from build123d import *

# Parameters (mm, degrees)
PAD012_DEPTH           = 5
LINEARPATTERN002_COUNT = 6
LINEARPATTERN002_PITCH = 15
SKETCH031_R            = 1.25
POCKET011_DEPTH        = 12
CHAMFER004_SIZE        = 1
FILLET004_R            = 3
FILLET005_R            = 1


with BuildPart() as part:
    # Sketch029 → Pad012 (new body, symmetric)
    with BuildSketch(Plane.YZ):
        Polygon((-18, 0), (93, 0), (85, 30), (-10, 30), align=None)
    extrude(amount=PAD012_DEPTH, both=True)

    # Sketch030 → Groove (revolve, cut)
    with BuildSketch(Plane.YZ):
        Polygon((0, 0), (1.8, 0), (1.8, 19.3), (2.5, 20), (2.5, 30), (0, 30), align=None)
    groove = revolve(axis=Axis((0, 0, 0), (0, 0, 1)), mode=Mode.SUBTRACT)

    # LinearPattern002: Groove ×6
    with Locations(*[(0, i * LINEARPATTERN002_PITCH, 0) for i in range(1, LINEARPATTERN002_COUNT)]):
        add(groove, mode=Mode.SUBTRACT)

    # Sketch031 → Pocket011 (cut)
    with BuildSketch(Plane.XY):
        with Locations((0, 85)):
            Circle(SKETCH031_R)
        with Locations((0, -10)):
            Circle(SKETCH031_R)
    extrude(amount=POCKET011_DEPTH, mode=Mode.SUBTRACT)

    # Chamfer004
    chamfer004_edges = [part.edges().sort_by_distance(p)[0] for p in [
        (0, -2.5, 30),
        (0, 12.5, 30),
        (0, 27.5, 30),
        (0, 42.5, 30),
        (0, 57.5, 30),
        (0, 72.5, 30),
    ]]
    chamfer(chamfer004_edges, length=CHAMFER004_SIZE)

    # Fillet004
    fillet004_edges = [part.edges().sort_by_distance(p)[0] for p in [
        (0, -10, 30),
        (0, 85, 30),
    ]]
    fillet(fillet004_edges, radius=FILLET004_R)

    # Fillet005
    fillet005_edges = [part.edges().sort_by_distance(p)[0] for p in [
        (5, -9.522873, 29.378967),
        (-5, 37.5, 30),
    ]]
    fillet(fillet005_edges, radius=FILLET005_R)


solid = part.part
Verification items for the finished model (mm, model axes). A direction names the side the tool comes from. Round coordinates to 2 decimals unless told otherwise and drop trailing zeros. Loops run counter-clockwise (first coordinate to the right, second up) from the corner with the lowest first, then second, coordinate; pieces in that order, holes last. Notation, with made-up numbers: (83, 81) - (106, 81) arc R23 cw to (106, 118) - close; hole circle Ø11 at (-37, 58). An arc over 180 degrees is marked (long way). Answer in a Markdown table with one row per item. Add a question column.
Q1. Section check B-B on z = 10. State how many separate pieces and enclosed holes the cut face has, plus the area to 3 significant figures.
Q2. Release check for a two-part mould opening along X. For faces 4 (the face through (0.056, -14.245, 14.081)), 5 (the face through (-4.7, 88.97, 14.01)), 6 (the face through (-0.1, 12.5, 24.6)), 7 (the face through (5, 37, 15)) record: pulls with the +X half, pulls with the -X half, needs draft (parallel to the pull), parting line crosses it, or undercut.
Q3. Material ranges on line 1 (X direction, y = 0, z = 19); line 2 (X direction, y = 60, z = 25.5); line 3 (Y direction, x = 3.5, z = 23), recorded low to high.
Q4. Gauge pin test, flat ends, axial feed: pin 1 (6 mm diameter, centred on x = 0, y = 30, fed in from +Z); pin 2 (4.5 mm diameter, centred on x = 0, y = 30, fed in from +Z); pin 3 (2 mm diameter, centred on x = -1, z = 12.5, fed in from -Y). Record the tip position at first contact, or that the pin passes through.
Q5. Section check A-A on y = 15. Enter the section's corners in (x, z), plus the area to 3 significant figures.
Q6. Tool access check on faces 1 (the face through (0.96, 47.31, 24.56)), 2 (the face through (0.672, -8.946, 5.916)), 3 (the face through (1.095, 73.572, 9.785)). Record the directions out of +Z, -Z, +X, -X, +Y, -Y that give a thin tool (end or side, any length) a straight path to the whole face; none if there is none.
Found:
| question | item | result |
|---|---|---|
| 1 | separate pieces | 1 |
| 1 | enclosed holes | 8 |
| 1 | area | 985 mm² |
| 2 | face 4 | needs draft |
| 2 | face 5 | pulls with the -X half |
| 2 | face 6 | undercut |
| 2 | face 7 | pulls with the +X half |
| 3 | line 1 | x = -5 to -1.8, 1.8 to 5 |
| 3 | line 2 | x = -5 to -2.5, 2.5 to 5 |
| 3 | line 3 | y = -11.87 to 86.87 |
| 4 | pin 1 | stops at z = 29.5 |
| 4 | pin 2 | stops at z = 19.75 |
| 4 | pin 3 | stops at y = -14.93 |
| 5 | outline | (-5, 0) - (-1.8, 0) - (-1.8, 19.3) - (-2.5, 20) - (-2.5, 29) - (-3.5, 30) - (-4, 30) arc R1 ccw to (-5, 29) - close; (1.8, 0) - (5, 0) - (5, 29) arc R1 ccw to (4, 30) - (3.5, 30) - (2.5, 29) - (2.5, 20) - (1.8, 19.3) - close |
| 5 | area | 176 mm² |
| 6 | face 1 | +Z |
| 6 | face 2 | -Z |
| 6 | face 3 | +Z, -Z |
